```python
from build123d import *

# Parameters (mm, degrees)
F0_R     = 2.6035
F0_W     = 2.7432
F0_H     = 2.7432
F1_DEPTH = 0.508
F2_W     = 3.681906
F2_H     = 3.681906
F2_W_2   = 2.7432
F2_H_2   = 2.7432
F3_DEPTH = 12.0396


with BuildPart() as f1:
    # F0 (on Top) → F1 (new body)
    with BuildSketch(Plane.XY):
        Circle(F0_R)
        Rectangle(F0_W, F0_H, mode=Mode.SUBTRACT)
    extrude(amount=F1_DEPTH)

    # F2 (on face) → F3 (join)
    with BuildSketch(Plane.XY.offset(0.508)):
        Rectangle(F2_W, F2_H)
        Rectangle(F2_W_2, F2_H_2, mode=Mode.SUBTRACT)
    extrude(amount=F3_DEPTH)


solid = f1.part
```
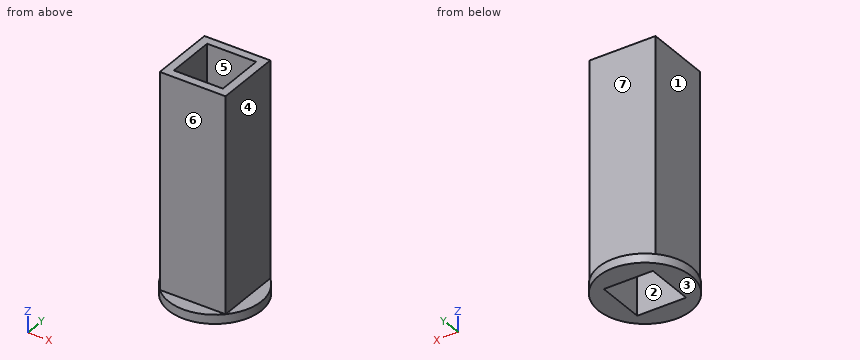
Can you work these out from the model? Positions are in its coordinate system, mm. Face numbers are marked on the shaded views. A direction names the side the tool comes from. Round coordinates to 2 decimals unless told otherwise and drop trailing zeros. Loops run counter-clockwise (first coordinate to the right, second up) from the corner with the lowest first, then second, coordinate; pieces in that order, holes last. Notation, with made-up numbers: M 69,57.5 L 79,57.5 A18 ccw 79,66.5 Z; hole C 3,-16 d5. An arc over 180 degrees is marked long. Answer as a JSON object with one key per item and string values. Group by question number.
Q1. We'd pull the mould along Y, two halves only. Please class the marked faces 5, 6 and 7: +Y half, -Y half, draft (parallel to the pull), parting line (faces both ways), or undercut.
Q2. On a 3-axis mill with a long thin cutter (end or side, diameter ignored), from which of +Z, -Z, +X, -X, +Y, -Y can I reach the whole of each face in a straight line? I mean the marked faces 1, 2, 3 and 4. Say none if no direction works.
Q3. Imagine slicing it at A-A, the plane y = 0. Please give me the cut outline in (x, z).
Q4. Imagine slicing it at D-D, the plane y = -1.55. Please give me the cut outline in (x, z), then the cut area to 3 significant figures.
Q5. Please list where these lines run through material, in increasing order: L1, parallel to Y at x = 0.2, z = 8.5; L2, parallel to Z at x = -0.65, y = -2.35.
Q6. Imagine slicing it at B-B, the plane z = 6.25. Please give me the cut outline in (x, y).
Q7. Will these pins go through, and if not, where does the flat tip stop? pin 1 (3 mm diameter, centred on y = 0.5, z = 8, fed in from +X); pin 2 (0.8 mm diameter, centred on x = 0.5, z = 6.5, fed in from -Y); pin 3 (1.4 mm diameter, centred on x = 0.5, z = 3.5, fed in from +Y).
Findings:
{
 "1": {"face 5": "undercut", "face 6": "-Y half", "face 7": "+Y half"},
 "2": {"face 1": "+Z, -X, +Y, -Y", "face 2": "+Z, -Z", "face 3": "-Z, +X, -X, +Y, -Y", "face 4": "+Z, +X, +Y, -Y"},
 "3": {"outline": "M -2.6,0 L -1.37,0 L -1.37,12.55 L -1.84,12.55 L -1.84,0.51 L -2.6,0.51 Z; M 1.37,0 L 2.6,0 L 2.6,0.51 L 1.84,0.51 L 1.84,12.55 L 1.37,12.55 Z"},
 "4": {"outline": "M -2.09,0 L 2.09,0 L 2.09,0.51 L 1.84,0.51 L 1.84,12.55 L -1.84,12.55 L -1.84,0.51 L -2.09,0.51 Z", "area": "46.5 mm2"},
 "5": {"L1": "y = -1.84 to -1.37, 1.37 to 1.84", "L2": "z = 0 to 0.51"},
 "6": {"outline": "M -1.84,-1.84 L 1.84,-1.84 L 1.84,1.84 L -1.84,1.84 Z; hole M -1.37,-1.37 L 1.37,-1.37 L 1.37,1.37 L -1.37,1.37 Z"},
 "7": {"pin 1": "stops at x = 1.84", "pin 2": "stops at y = -1.84", "pin 3": "stops at y = 1.84"}
}
